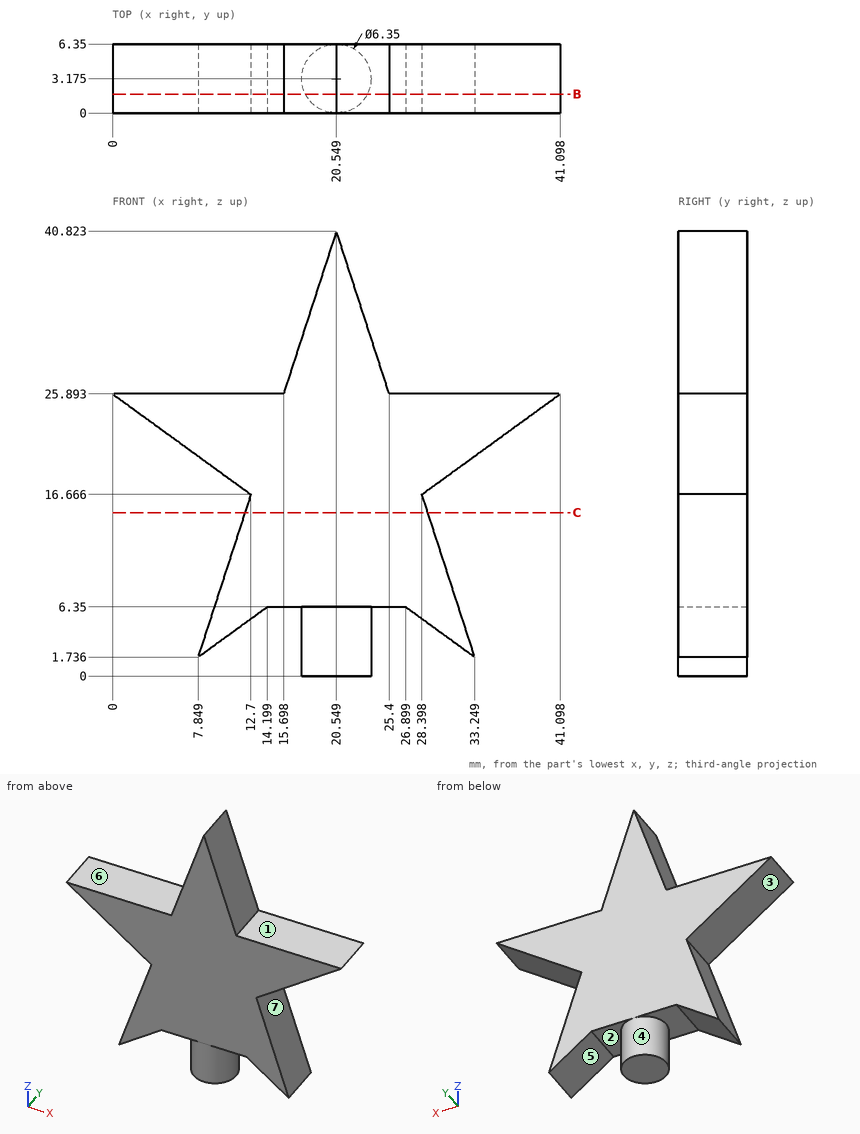
Geometry: see drawing. Coordinates: mm, zero at the bounding-box minimum. A direction names the side the tool comes from. Round coordinates to 2 decimals unless told otherwise and drop trailing zeros. Write each loop counter-clockwise with the first axis right and the second up, starting at its lowest first coordinate (ties: lowest second). Pieces come first, ordered by that corner, then holes.
1) Contact query for flat-ended pins moving along their axis: P1, Ø1, axis at y = 2, z = 18.5, coming from the -X side; P2, Ø2, axis at x = 35.5, y = 1.5, coming from the +Z side; P3, Ø2, axis at y = 4.5, z = 22.5, coming from the -X side (1 decimal). Output: stop coordinate, or through.
2) Cut plane C-C (z = 15). Return the cut outline in (x, y).
3) Ray query, L1, parallel to X at y = 1, z = 5 (1 decimal); L2, parallel to Z at x = 15, y = 2.5; L3, parallel to X at y = 6, z = 34.5 (1 decimal). Return the intervals inside material, ascending.
4) Reachability of the marked faces 4, 5, 6 and 7 from +Z, -Z, +X, -X, +Y, -Y: full face, straight path, thin tool, end or side. Return the list, or none.
5) Draft query along X for the marked faces 1, 2 and 3. Return one class per face: pulls with the +X half, pulls with the -X half, needs draft (parallel to the pull), parting line crosses it, or undercut.
6) Cut plane B-B (y = 1.75). Return the cut outline in (x, z).
Geometry says:
1. P1: stops at x = 9.49
1. P2: stops at z = 25.89
1. P3: stops at x = 3.3
2. outline: (12.16, 0) - (28.94, 0) - (28.94, 6.35) - (12.16, 6.35) - close
3. L1: x = 8.9 to 12.3, 18.2 to 22.9, 28.8 to 32.2
3. L2: z = 6.35 to 25.89
3. L3: x = 18.5 to 22.6
4. face 4: -Z
4. face 5: -Z, +Y, -Y
4. face 6: +Z, -X, +Y, -Y
4. face 7: +X, +Y, -Y
5. face 1: needs draft
5. face 2: undercut
5. face 3: pulls with the -X half
6. outline: (0, 25.89) - (12.7, 16.67) - (7.85, 1.74) - (14.2, 6.35) - (17.71, 6.35) - (17.71, 0) - (23.39, 0) - (23.39, 6.35) - (26.9, 6.35) - (33.25, 1.74) - (28.4, 16.67) - (41.1, 25.89) - (25.4, 25.89) - (20.55, 40.82) - (15.7, 25.89) - close
